Source: CAD feature listing. Evaluate the final solid. Frame: model axes, mm. Give positions to 0.01 mm unless a question says otherwise; leave off trailing zeros. Put each result on its own line as item: value.
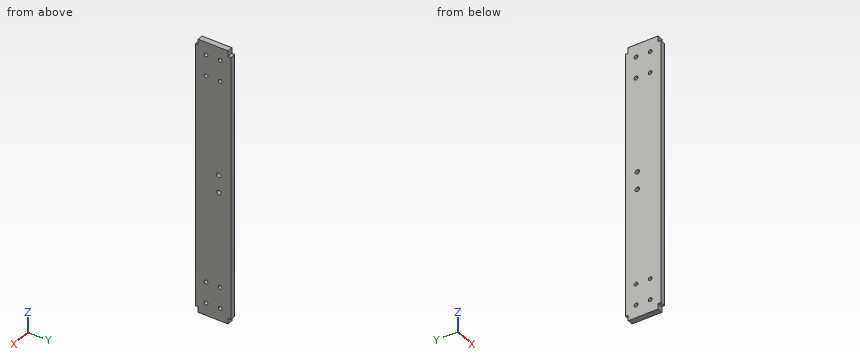
```python
from build123d import *

# Parameters (mm, degrees)
SKETCH1_W              = 300
SKETCH1_H              = 40
BOSS_EXTRUDE1_DEPTH    = 6.35
SKETCH2_W              = 6.35
SKETCH2_H              = 33.65
BOSS_EXTRUDE2_DEPTH    = 6.35
F_10_CLEARANCE_HOLE1_D = 4.9784
F_8_CLEARANCE_HOLE1_D  = 4.3053


with BuildPart() as part:
    # Sketch1 → Boss-Extrude1 (new body)
    with BuildSketch(Plane(origin=(0, 0, 0), x_dir=(0, 0, -1), z_dir=(1, 0, 0))):
        Rectangle(SKETCH1_W, SKETCH1_H)
    extrude(amount=BOSS_EXTRUDE1_DEPTH)

    # Sketch2 → Boss-Extrude2 (add)
    with BuildSketch(Plane(origin=(6.35, 0, 0), x_dir=(0, 0, -1), z_dir=(1, 0, 0))):
        with Locations((-153.175, 0)):
            Rectangle(SKETCH2_W, SKETCH2_H)
        with Locations((153.175, 0)):
            Rectangle(SKETCH2_W, SKETCH2_H)
    extrude(amount=-BOSS_EXTRUDE2_DEPTH)

    # #10 Clearance Hole1 (through all)
    with Locations(Plane(origin=(6.35, 0, 0), x_dir=(0, 0, -1), z_dir=(1, 0, 0))):
        with Locations((-10, 6.5), (10, 6.5)):
            Hole(F_10_CLEARANCE_HOLE1_D / 2)

    # #8 Clearance Hole1 (through all)
    with Locations(Plane(origin=(6.35, 0, 0), x_dir=(0, 0, -1), z_dir=(1, 0, 0))):
        with Locations((-142, 8), (-118, 8), (-118, -8), (-142, -8), (118, 8), (142, 8), (142, -8), (118, -8)):
            Hole(F_8_CLEARANCE_HOLE1_D / 2)


solid = part.part
```
1) Pin query (flat end, axial travel): P1, Ø1.6, axis at x = 4, y = -18, coming from the -Z side; P2, Ø3, axis at x = 2.5, z = -152.5, coming from the +Y side (3 decimals); P3, Ø3, axis at x = 4, z = -152, coming from the -Y side (3 decimals). Return the tip coordinate at first contact, or that it passes through.
Check result:
P1: z = -150
P2: y = 16.825
P3: y = -16.825
2) Material intervals for line 1 along Y through (x, z) = (1.75, 142); line 2 along Y through (x, z) = (3, -10); line 3 along Z through (x, y) = (3.25, -17), sorted ascending. Write a range as [from, to].
Check result:
line 1: [-20, -10.15], [-5.85, 5.85], [10.15, 20]
line 2: [-20, 4.01], [8.99, 20]
line 3: [-150, 150]
3) Section query A-A, the plane x = 3. State how many separate pieces and enclosed holes the cut face has, plus the area to 3 significant figures.
Check result:
separate pieces: 1
enclosed holes: 10
area: 12,300 mm²
